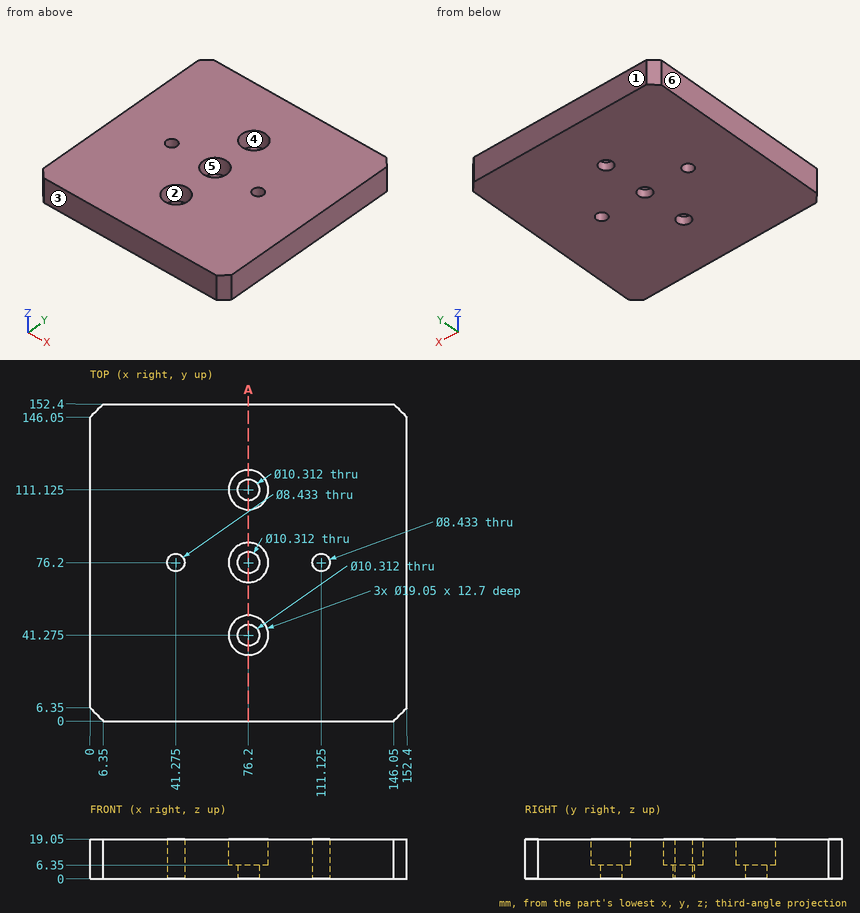
Geometry check sheet. Reference: drawing and pictorial views, mm from the part's lowest x, y, z. A direction names the side the tool comes from. Give positions to 0.01 mm unless a question says otherwise; leave off trailing zeros. Use CSV: the item, a comma, the result in double quotes. Start each with the question number.
1) Sectioned sample at A-A, the plane x = 76.2. Give the number of separate pieces and of enclosed holes in the cut face, plus the area to 3 significant figures.
2) Mould release check, pull along Y, two halves, no side actions. Record for the marked faces 3, 4, 5 and 6: released by +Y, released by -Y, zero draft, split by the parting line, or undercut.
3) Material ranges on line 1 (X direction, y = 73, z = 13.5); line 2 (Y direction, x = 71.5, z = 3) (1 decimal); line 3 (X direction, y = 115, z = 16.25), recorded low to high. Write a range as from..to.
4) Go/stop test with flat-tipped pins: P1, Ø5.5, axis at x = 78, y = 109, coming from the +Z side; P2, Ø5, axis at x = 111.125, y = 76.2, coming from the -Z side. Record where each tip stops, or that it passes through.
5) Set-up check for the marked faces 1 and 2: record each of +Z, -Z, +X, -X, +Y, -Y from which the full face is reachable in a straight line by a thin tool's end or side.
Recorded:
1,separate pieces,"4"
1,enclosed holes,"0"
1,area,"1,980 mm2"
2,face 3,"released by -Y"
2,face 4,"undercut"
2,face 5,"undercut"
2,face 6,"zero draft"
3,line 1,"0..38.53, 44.02..67.23, 85.17..108.38, 113.87..152.4"
3,line 2,"0..39.2, 43.4..74.1, 78.3..109, 113.2..152.4"
3,line 3,"0..67.5, 84.9..152.4"
4,P1,"z = 6.35"
4,P2,"through"
5,face 1,"+Z, -Z, +X, -X, +Y"
5,face 2,"+Z"
